Can you work these out from the drawing? Everything is in mm from the part's minimum corner. A direction names the side the tool comes from. Coordinates: 2 decimals unless noted, no trailing zeros. Loops run counter-clockwise (first coordinate to the right, second up) from the corner with the lowest first, then second, coordinate; pieces in that order, holes last. Notation, with made-up numbers: (-40, 22) - (-9, 22) arc R15 ccw to (-9, 29) - close; hole circle Ø7 at (39.5, -13). An arc over 180 degrees is marked (long way). Put each result on its own line as item: value. Start each with the question number.
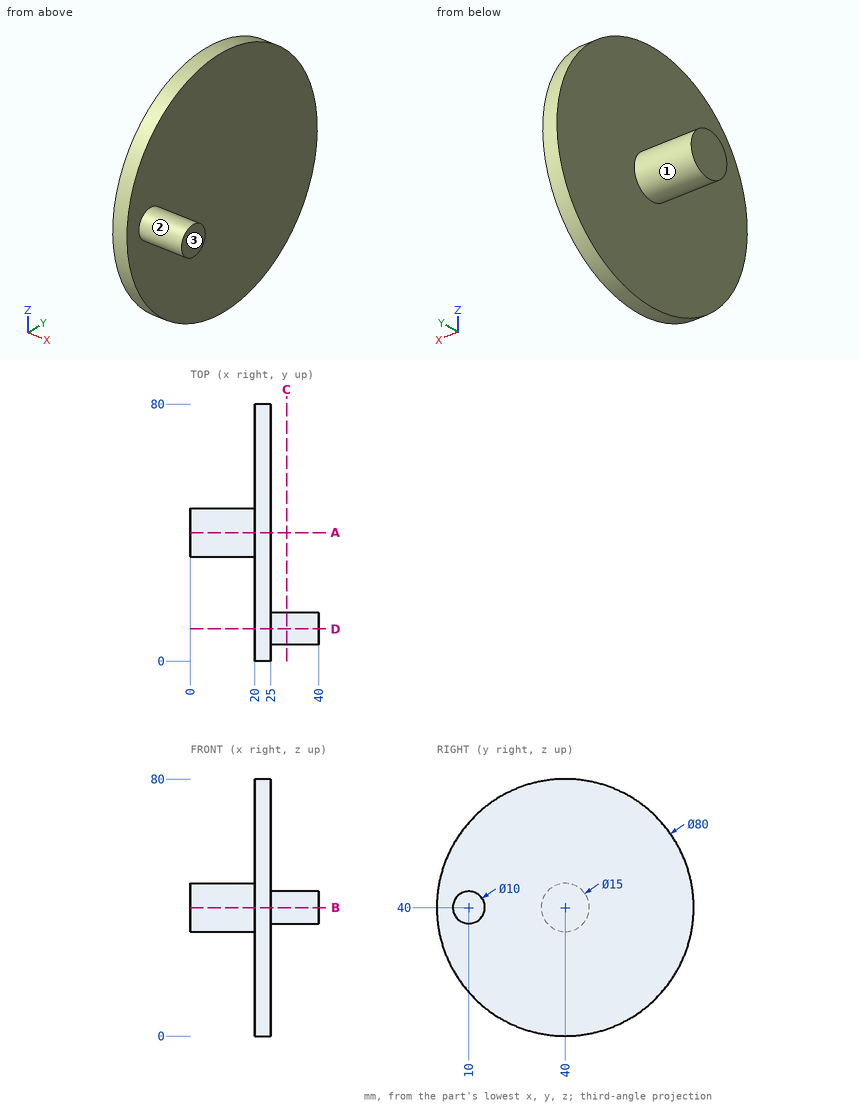
Q1. I want a section at A-A on y = 40. List the corners of the cut face in (x, z) for me, and give its area (3 significant figures).
Q2. I want a section at B-B on z = 40. List the corners of the cut face in (x, y) for me.
Q3. On a 3-axis mill with a long thin cutter (end or side, diameter ignored), from which of +Z, -Z, +X, -X, +Y, -Y can I reach the whole of each face in a straight line? I mean the marked faces 1, 2 and 3. Say none if no direction works.
Q4. I want a section at D-D on y = 10. List the corners of the cut face in (x, z) for me.
Q5. Please list where these lines run through material, in increasing order: line 1 along X through (y, z) = (47.5, 14.5); line 2 along Z through (x, y) = (23, 60); line 3 along Z through (x, y) = (2.5, 45). Write a range as [from, to].
Q6. I want a section at C-C on x = 30. List the corners of the cut face in (y, z) for me.
Q7. Will these pins go through, and if not, where does the flat tip stop? pin 1 (5 mm diameter, centred on x = 4, z = 38.5, fed in from -Y); pin 2 (4 mm diameter, centred on x = 25.5, y = 71, fed in from +Z); pin 3 (5 mm diameter, centred on y = 55, z = 67, fed in from -X).
Calculated:
1. outline: (0, 32.5) - (20, 32.5) - (20, 0) - (25, 0) - (25, 80) - (20, 80) - (20, 47.5) - (0, 47.5) - close
1. area: 700 mm2
2. outline: (0, 32.5) - (20, 32.5) - (20, 0) - (25, 0) - (25, 5) - (40, 5) - (40, 15) - (25, 15) - (25, 80) - (20, 80) - (20, 47.5) - (0, 47.5) - close
3. face 1: -X
3. face 2: +X
3. face 3: +Z, -Z, +X, +Y, -Y
4. outline: (20, 13.54) - (25, 13.54) - (25, 35) - (40, 35) - (40, 45) - (25, 45) - (25, 66.46) - (20, 66.46) - close
5. line 1: [20, 25]
5. line 2: [5.36, 74.64]
5. line 3: [34.41, 45.59]
6. outline: circle Ø10 at (10, 40)
7. pin 1: y = 32.5
7. pin 2: z = 67.48
7. pin 3: x = 20
